Input: part model. Units: mm. Frame: model coordinates. Coordinates: 2 decimals unless noted, no trailing zeros. Write each loop counter-clockwise with the first axis right and the second up, starting at its lowest first coordinate (ties: lowest second). Pieces come first, ordered by that corner, then holes. Notation, with made-up numbers: M 49,77 L 107,77 A25 ccw 107,99 Z; hole C 83,36 d4. An arc over 180 degrees is marked long. Write each question's results on one line, items separated by ' | '. Start each with the question number.
1. Section query B-B, the plane x = 166.5. Output: boundary loops of the cut face in (y, z), and give its area (3 significant figures).
2. Section query C-C, the plane z = 27. Output: boundary loops of the cut face in (x, y), and give its area (4 significant figures).
3. First-contact query: pin 1 (0.6 mm diameter, centred on y = -0.5, z = 22.5, fed in from +X); pin 2 (1.2 mm diameter, centred on x = 553, y = 0.5, fed in from +Z). Flat tips, straight axial feed; report the tip coordinate or a pass-through.
4. Section query A-A, the plane y = 0.55. Output: boundary loops of the cut face in (x, z), and give its area (3 significant figures).
5. Section query D-D, the plane z = 5.5. Output: boundary loops of the cut face in (x, y), and give its area (3 significant figures).
6. Ray query, probe 1 along X at (y, z) = (0.7, 37.5); probe 2 along Y at (x, z) = (217.5, 34.5); probe 3 along X at (y, z) = (0.25, 10.5). Return the intervals inside material, ascending.
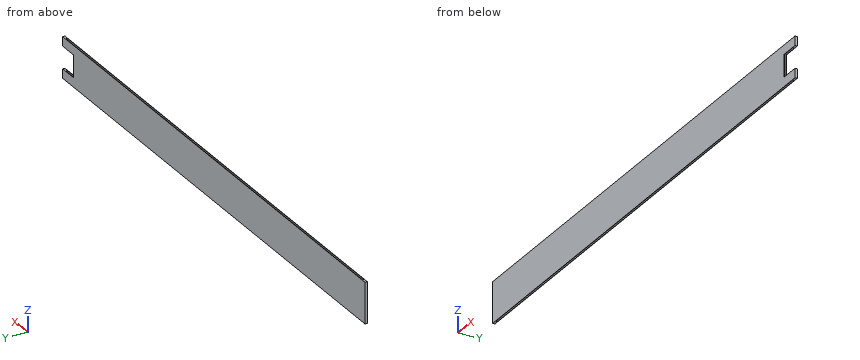
```python
from build123d import *

# Parameters (mm, degrees)
F0_W     = 560
F0_H     = 44
F1_DEPTH = 0.5
F2_W     = 5
F2_H     = 44
F3_DEPTH = 1.5
F4_W     = 560
F4_H     = 44
F5_DEPTH = 0.5
F6_W     = 20
F6_H     = 24
F7_DEPTH = 2.501


with BuildPart() as f1:
    # F0 (on Front) → F1 (new body)
    with BuildSketch(Plane.XZ):
        with Locations((280, 22)):
            Rectangle(F0_W, F0_H)
    extrude(amount=F1_DEPTH)

    # F2 (on face) → F3 (join)
    with BuildSketch(Plane(origin=(0, 0, 0), x_dir=(-1, 0, 0), z_dir=(0, 1, 0))):
        with Locations((-557.5, 22)):
            Rectangle(F2_W, F2_H)
        with Locations((-2.5, 22)):
            Rectangle(F2_W, F2_H)
    extrude(amount=F3_DEPTH)

    # F4 (on face) → F5 (join)
    with BuildSketch(Plane(origin=(0, 1.5, 0), x_dir=(-1, 0, 0), z_dir=(0, 1, 0))):
        with Locations((-280, 22)):
            Rectangle(F4_W, F4_H)
    extrude(amount=F5_DEPTH)

    # F6 (on face) → F7 (cut, through all)
    with BuildSketch(Plane(origin=(0, 2, 0), x_dir=(-1, 0, 0), z_dir=(0, 1, 0))):
        with Locations((-550, 22)):
            Rectangle(F6_W, F6_H)
    extrude(amount=-F7_DEPTH, mode=Mode.SUBTRACT)


solid = f1.part
```
Answer:
1) outline: M -0.5,0 L 0,0 L 0,44 L -0.5,44 Z; M 1.5,0 L 2,0 L 2,44 L 1.5,44 Z | area: 44.0 mm^2
2) outline: M 0,-0.5 L 540,-0.5 L 540,0 L 5,0 L 5,1.5 L 540,1.5 L 540,2 L 0,2 Z | area: 547.5 mm^2
3) pin 1: x = 540 | pin 2: z = 44
4) outline: M 0,0 L 5,0 L 5,44 L 0,44 Z; M 555,0 L 560,0 L 560,10 L 555,10 Z; M 555,34 L 560,34 L 560,44 L 555,44 Z | area: 320 mm^2
5) outline: M 0,-0.5 L 560,-0.5 L 560,2 L 0,2 Z; hole M 5,0 L 555,0 L 555,1.5 L 5,1.5 Z | area: 575 mm^2
6) probe 1: 0 to 5, 555 to 560 | probe 2: -0.5 to 0, 1.5 to 2 | probe 3: 0 to 5
